Could you check a few things on this model? Use its own coordinates, in mm. Face numbers are marked on the shaded views. A direction names the side the tool comes from. Round coordinates to 2 decimals unless told otherwise and drop trailing zeros. Loops run counter-clockwise (first coordinate to the right, second up) from the corner with the lowest first, then second, coordinate; pieces in that order, holes last.
from build123d import *

# Parameters (mm, degrees)
SKETCH1_R           = 4.7625
SKETCH1_R_2         = 1.905
BOSS_EXTRUDE1_DEPTH = 6.35
FILLET1_R           = 3.81
FILLET2_R           = 3.81


with BuildPart() as part:
    # Sketch1 → Boss-Extrude1 (new body)
    # profile 1 of 10: a face of its own
    with BuildSketch(Plane.XY):
        with Locations((106.189208713, 23.71)):
            Circle(SKETCH1_R)
        with Locations((106.189208713, 23.71)):
            Circle(SKETCH1_R_2, mode=Mode.SUBTRACT)
    # profile 2 of 10: a face of its own
    with BuildSketch(Plane.XY):
        with BuildLine():
            Line((87.880964772, -0.786362752), (104.53862394, 19.242676846))
            ThreePointArc((104.53862394, 19.242676846), (103.143914747, 20.048362263), (102.097532116, 21.272872823))
            Line((102.097532116, 21.272872823), (86.113888675, 2.054264483))
            Line((86.113888675, 2.054264483), (58.96261429, 18.093110387))
            ThreePointArc((58.96261429, 18.093110387), (58.389707875, 16.587746324), (57.347778506, 15.359444279))
            Line((57.347778506, 15.359444279), (82.443811077, 0.534674233))
            Line((82.443811077, 0.534674233), (58.194514032, -6.164197988))
            ThreePointArc((58.194514032, -6.164197988), (58.832358657, -7.4612961), (59.051708713, -8.89))
            ThreePointArc((59.051708713, -8.89), (59.048766191, -9.057388361), (59.039942261, -9.224569879))
            Line((59.039942261, -9.224569879), (84.017242402, -2.324586685))
            Line((84.017242402, -2.324586685), (75.126101157, -28.865420044))
            ThreePointArc((75.126101157, -28.865420044), (76.717900747, -29.111421646), (78.136663259, -29.873954045))
            Line((78.136663259, -29.873954045), (87.880964772, -0.786362752))
        make_face()
    # profile 3 of 10: a face of its own
    with BuildSketch(Plane.XY):
        with BuildLine():
            ThreePointArc((101.428860996, 23.566836206), (101.65338858, 25.161806453), (102.396731965, 26.590716294))
            Line((102.396731965, 26.590716294), (79.965447461, 33.770428593))
            ThreePointArc((79.965447461, 33.770428593), (79.967061643, 33.698854784), (79.967599745, 33.627264799))
            ThreePointArc((79.967599745, 33.627264799), (79.718583807, 32.107439852), (78.997576492, 30.746548504))
            Line((78.997576492, 30.746548504), (101.428860996, 23.566836206))
        make_face()
    # profile 4 of 10: a face of its own
    with BuildSketch(Plane.XY):
        with Locations((75.205099745, 33.627264799)):
            Circle(SKETCH1_R)
        with Locations((75.205099745, 33.627264799)):
            Circle(SKETCH1_R_2, mode=Mode.SUBTRACT)
    # profile 5 of 10: a face of its own
    with BuildSketch(Plane.XY):
        with BuildLine():
            ThreePointArc((72.434047253, 29.753936212), (71.301416872, 30.89913975), (70.615297221, 32.356391461))
            Line((70.615297221, 32.356391461), (57.060261204, 22.883328587))
            ThreePointArc((57.060261204, 22.883328587), (58.192891585, 21.738125049), (58.879011236, 20.280873338))
            Line((58.879011236, 20.280873338), (72.434047253, 29.753936212))
        make_face()
    # profile 6 of 10: a face of its own
    with BuildSketch(Plane.XY):
        with Locations((54.289208713, 19.01)):
            Circle(SKETCH1_R)
        with Locations((54.289208713, 19.01)):
            Circle(SKETCH1_R_2, mode=Mode.SUBTRACT)
    # profile 7 of 10: a face of its own
    with BuildSketch(Plane.XY):
        with BuildLine():
            ThreePointArc((55.876708713, 14.519871939), (54.289208713, 14.2475), (52.701708713, 14.519871939))
            Line((52.701708713, 14.519871939), (52.701708713, -4.399871939))
            ThreePointArc((52.701708713, -4.399871939), (54.289208713, -4.1275), (55.876708713, -4.399871939))
            Line((55.876708713, -4.399871939), (55.876708713, 14.519871939))
        make_face()
    # profile 8 of 10: a face of its own
    with BuildSketch(Plane.XY):
        with Locations((54.289208713, -8.89)):
            Circle(SKETCH1_R)
        with Locations((54.289208713, -8.89)):
            Circle(SKETCH1_R_2, mode=Mode.SUBTRACT)
    # profile 9 of 10: a face of its own
    with BuildSketch(Plane.XY):
        with BuildLine():
            ThreePointArc((58.400562122, -11.29378439), (57.364168417, -12.526760793), (55.976054927, -13.343757526))
            Line((55.976054927, -13.343757526), (71.093746335, -31.223480409))
            ThreePointArc((71.093746335, -31.223480409), (72.13014004, -29.990504006), (73.518253531, -29.173507273))
            Line((73.518253531, -29.173507273), (58.400562122, -11.29378439))
        make_face()
    # profile 10 of 10: a face of its own
    with BuildSketch(Plane.XY):
        with Locations((75.205099745, -33.627264799)):
            Circle(SKETCH1_R)
        with Locations((75.205099745, -33.627264799)):
            Circle(SKETCH1_R_2, mode=Mode.SUBTRACT)
    extrude(amount=BOSS_EXTRUDE1_DEPTH)

    # Fillet1
    # the kernel refuses this fillet: 3.81 mm, written as the material it adds along each edge
    with BuildSketch(Plane(origin=(58.96261429, 18.093110387, 0), x_dir=(0.8609971993913142, -0.5086096957789081, 0), z_dir=(0, 0, 1)), Plane(origin=(75.126101157, -28.865420044, 0), x_dir=(0.31764850444110154, 0.9482085359383406, 0), z_dir=(0, 0, 1)), Plane(origin=(79.965447461, 33.770428593, 0), x_dir=(0.9524031774112249, -0.30484124992691375, 0), z_dir=(0, 0, 1)), Plane(origin=(104.53862394, 19.242676846, 0), x_dir=(-0.6394318036990395, -0.7688478187640211, 0), z_dir=(0, 0, 1)), Plane(origin=(52.701708713, -4.399871939, 0), x_dir=(0, 1, 0), z_dir=(0, 0, 1)), Plane(origin=(57.060261204, 22.883328587, 0), x_dir=(0.8196709443644911, 0.572834655869059, 0), z_dir=(0, 0, 1))) as fillet1_piece_1:
        with BuildLine():
            CenterArc((2.169808125, 3.81), FILLET1_R, 219.022802565, 50.977197435)
            ThreePointArc((-0.790163513, 1.411111111), (-0.334744459, 0.739341932), (0, 0))
            Line((0, 0), (2.169808125, 0))
        make_face()
    extrude(amount=6.35)
    with BuildSketch(Plane(origin=(86.113888675, 2.054264483, 0), x_dir=(-0.8609971993913146, 0.5086096957789075, 0), z_dir=(0, 0, 1))) as fillet1_piece_2:
        with BuildLine():
            CenterArc((FILLET1_R * 0.85139484235, -FILLET1_R), FILLET1_R, 90, 80.821803005)
            Line((-FILLET1_R * 0.135802191515, -FILLET1_R * 0.840494463015), (0, 0))
            Line((0, 0), (FILLET1_R * 0.85139484235, 0))
        make_face()
    extrude(amount=6.35)
    with BuildSketch(Plane(origin=(102.097532116, 21.272872823, 0), x_dir=(-0.6394318036990395, -0.7688478187640211, 0), z_dir=(0, 0, 1)), Plane(origin=(78.997576492, 30.746548504, 0), x_dir=(0.9524031774112243, -0.3048412499269152, 0), z_dir=(0, 0, 1)), Plane(origin=(58.879011236, 20.280873338, 0), x_dir=(0.819670944364491, 0.5728346558690592, 0), z_dir=(0, 0, 1)), Plane(origin=(73.518253531, -29.173507273, 0), x_dir=(-0.6456608303485428, 0.7636243134903644, 0), z_dir=(0, 0, 1)), Plane(origin=(59.039942261, -9.224569879, 0), x_dir=(0.9638966585389959, 0.2662766074167205, 0), z_dir=(0, 0, 1)), Plane(origin=(57.347778506, 15.359444279, 0), x_dir=(0.8609971993913154, -0.5086096957789064, 0), z_dir=(0, 0, 1))) as fillet1_piece_3:
        with BuildLine():
            CenterArc((2.169808125, -3.81), FILLET1_R, 90, 50.977197435)
            ThreePointArc((-0.790163513, -1.411111111), (-0.334744459, -0.739341932), (0, 0))
            Line((0, 0), (2.169808125, 0))
        make_face()
    extrude(amount=6.35)
    with BuildSketch(Plane(origin=(101.428860996, 23.566836206, 0), x_dir=(0.19934053923435113, -0.9799302778349887, 0), z_dir=(0, 0, 1)), Plane(origin=(72.434047253, 29.753936212, 0), x_dir=(0.9002818811258162, -0.4353074023222692, 0), z_dir=(0, 0, 1)), Plane(origin=(58.400562122, -11.29378439, 0), x_dir=(0.3508244107521176, 0.9364412596743211, 0), z_dir=(0, 0, 1)), Plane(origin=(58.194514032, -6.164197988, 0), x_dir=(-0.7032685796981372, 0.7109242609514496, 0), z_dir=(0, 0, 1)), Plane(origin=(55.876708713, 14.519871939, 0), x_dir=(0.8725214911102023, 0.48857573369010987, 0), z_dir=(0, 0, 1)), Plane(origin=(71.093746335, -31.223480409, 0), x_dir=(-0.3508244107521106, -0.9364412596743238, 0), z_dir=(0, 0, 1))) as fillet1_piece_4:
        with BuildLine():
            CenterArc((2.264191284, -3.754677766), FILLET1_R, 99.775790965, 50.977197435)
            Line((-1.060115597, -1.893204221), (0, 0))
            ThreePointArc((0, 0), (0.808639744, -0.069152792), (1.617279489, 0))
        make_face()
    extrude(amount=6.35)
    with BuildSketch(Plane(origin=(84.017242402, -2.324586685, 0), x_dir=(-0.3176485044411025, -0.9482085359383404, 0), z_dir=(0, 0, 1))) as fillet1_piece_5:
        with BuildLine():
            CenterArc((FILLET1_R * 1.8792860539, -FILLET1_R), FILLET1_R, 90, 123.963598679)
            Line((FILLET1_R * 1.04989338062, -FILLET1_R * 1.55866608409), (0, 0))
            Line((0, 0), (FILLET1_R * 1.8792860539, 0))
        make_face()
    extrude(amount=6.35)
    with BuildSketch(Plane(origin=(55.876708713, -4.399871939, 0), x_dir=(0.8725214911102017, -0.488575733690111, 0), z_dir=(0, 0, 1)), Plane(origin=(70.615297221, 32.356391461, 0), x_dir=(-0.09933921507111794, 0.9950536268709613, 0), z_dir=(0, 0, 1)), Plane(origin=(102.396731965, 26.590716294, 0), x_dir=(0.7313016231106118, 0.682054203150882, 0), z_dir=(0, 0, 1)), Plane(origin=(78.136663259, -29.873954045, 0), x_dir=(0.6721369745474647, -0.740426827881176, 0), z_dir=(0, 0, 1)), Plane(origin=(55.976054927, -13.343757526, 0), x_dir=(-0.9817328385571232, -0.1902646412199953, 0), z_dir=(0, 0, 1)), Plane(origin=(52.701708713, 14.519871939, 0), x_dir=(-0.8725214911102018, 0.48857573369011076, 0), z_dir=(0, 0, 1))) as fillet1_piece_6:
        with BuildLine():
            CenterArc((2.264191284, 3.754677766), FILLET1_R, 209.2470116, 50.977197435)
            Line((-1.060115597, 1.893204221), (0, 0))
            ThreePointArc((0, 0), (0.808639744, 0.069152792), (1.617279489, 0))
        make_face()
    extrude(amount=6.35)
    with BuildSketch(Plane(origin=(82.443811077, 0.534674233, 0), x_dir=(-0.9638966585389961, -0.2662766074167203, 0), z_dir=(0, 0, 1))) as fillet1_piece_7:
        with BuildLine():
            CenterArc((FILLET1_R * 2.35504725068, -FILLET1_R), FILLET1_R, 90, 133.985910602)
            Line((FILLET1_R * 1.63553665117, -FILLET1_R * 1.69448145921), (0, 0))
            Line((0, 0), (FILLET1_R * 2.35504725068, 0))
        make_face()
    extrude(amount=6.35)
    with BuildSketch(Plane(origin=(87.880964772, -0.786362752, 0), x_dir=(-0.3176485044411054, -0.9482085359383393, 0), z_dir=(0, 0, 1))) as fillet1_piece_8:
        with BuildLine():
            CenterArc((FILLET1_R * 0.187404040861, FILLET1_R), FILLET1_R, 248.771312287, 21.228687713)
            Line((-FILLET1_R * 0.174687293783, FILLET1_R * 0.0678573792733), (0, 0))
            Line((0, 0), (FILLET1_R * 0.187404040861, 0))
        make_face()
    extrude(amount=6.35)

    # Fillet2
    fillet2_edges = [part.edges().sort_by_distance(p)[0] for p in [
        (74.278682032, -28.792470042, 3.175),
        (59.113584062, 19.194358415, 3.175),
        (58.904928759, -10.316241556, 3.175),
        (56.72342156, 14.744855925, 3.175),
    ]]
    fillet(fillet2_edges, radius=FILLET2_R)


solid = part.part
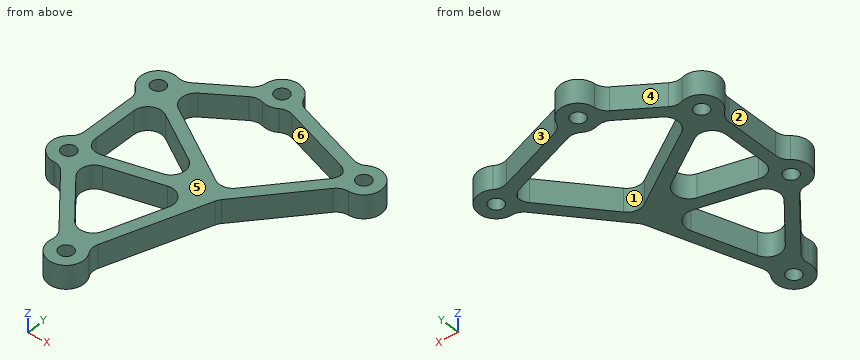
Item 1: If I drill on line 1 along Y through (x, z) = (54.5, 6); line 2 along Y through (x, z) = (75.5, 5.5); line 3 along Y through (x, z) = (70, 1), over which ranges is the centre line in solid material (lowest first)?
Results list:
line 1: y = -13.65 to -10.78, -7 to 17.12, 20.9 to 23.77
line 2: y = -38.38 to -35.51, -31.75 to -25.8, -4.68 to -0.85, 4.49 to 8.32, 28.87 to 31.75, 35.51 to 38.38
line 3: y = -29.98 to -25.01, -6.2 to -2.9, 7.89 to 11.57, 28.05 to 32.41
Item 2: If we section it at B-B, the plane x = 85: Please give me the cut outline in (y, z), then the cut area to 3 significant figures.
Results list:
outline: (-9.39, 0) - (3.18, 0) - (3.18, 6.35) - (-9.39, 6.35) - close; (28.83, 0) - (32.16, 0) - (32.16, 6.35) - (28.83, 6.35) - close
area: 101 mm2
Item 3: If we section it at C-C, the plane z = 1.5: Count the separate pieces of the cut face and the enclosed holes in it, then the cut area to 3 significant figures.
Results list:
separate pieces: 1
enclosed holes: 8
area: 990 mm2
Item 4: For the marked faces 1, 2 and 3, which set-ups out of +Z, -Z, +X, -X, +Y, -Y let a thin tool reach every point of the face, with its end or its side?
Results list:
face 1: +Z, -Z
face 2: +Z, -Z, -X
face 3: +Z, -Z, +Y
Item 5: Will these pins go through, and if not, where does the flat tip stop? pin 1 (1.9 mm diameter, centred on y = 3.5, z = 3.5, fed in from +X); pin 2 (5 mm diameter, centred on x = 54.29, y = 19.01, fed in from +Z); pin 3 (2 mm diameter, centred on y = -29.5, z = 4, fed in from -X); pin 4 (1.5 mm diameter, centred on y = 20, z = 5, fed in from +X).
Results list:
pin 1: stops at x = 92.24
pin 2: stops at z = 6.35
pin 3: stops at x = 68.79
pin 4: stops at x = 109.92
Item 6: If we section it at A-A, the plane y = -18.5: Please give me the cut outline in (x, z), then the cut area to 3 significant figures.
Results list:
outline: (60.34, 0) - (64.49, 0) - (64.49, 6.35) - (60.34, 6.35) - close; (78.6, 0) - (81.95, 0) - (81.95, 6.35) - (78.6, 6.35) - close
area: 47.7 mm2
Item 7: We'd pull the mould along X, two halves only. Please class the marked faces 4, 5 and 6: released by +X, released by -X, zero draft, split by the parting line, or undercut.
Results list:
face 4: released by -X
face 5: zero draft
face 6: undercut
